Source: CAD feature listing. Evaluate the final solid. Frame: model axes, mm. Give positions to 0.01 mm unless a question says otherwise; leave off trailing zeros. One line per question, with ' | ' between items. Start each with the question number.
(1) Section A-A, the plane y = 5. State how many separate pieces and enclosed holes the cut face has, plus the area to 3 significant figures.
(2) Ray query, line 1 (Y direction, x = -20, z = 1.1); line 2 (Y direction, x = 72, z = 1.7). Return the intervals inside material, ascending. Write a range as [from, to].
(3) Pin query (flat end, axial travel): pin 1 (1 mm diameter, centred on y = 4.5, z = 2, fed in from -X). Return the tip coordinate at first contact, or that it passes through.
```python
from build123d import *

# Parameters (mm, degrees)
SALIENTE_EXTRUIR1_DEPTH = 3


with BuildPart() as part:
    # Croquis1 → Saliente-Extruir1 (new body)
    with BuildSketch(Plane.XY):
        Polygon((-150, 2.5), (-165, 2.5), (-165, -7.5), (-150, -7.5), (150, -7.5), (165, -7.5), (165, 2.5), (150, 2.5), (147.707897557, 7.5), (145, 2.5), (142.707897557, 7.5), (140, 2.5), (137.707897557, 7.5), (135, 2.5), (132.707897557, 7.5), (130, 2.5), (127.707897557, 7.5), (125, 2.5), (122.707897557, 7.5), (120, 2.5), (117.707897557, 7.5), (115, 2.5), (112.707897557, 7.5), (110, 2.5), (107.707897557, 7.5), (105, 2.5), (102.707897557, 7.5), (100, 2.5), (97.707897557, 7.5), (95, 2.5), (92.707897557, 7.5), (90, 2.5), (87.707897557, 7.5), (85, 2.5), (82.707897557, 7.5), (80, 2.5), (77.707897557, 7.5), (75, 2.5), (72.707897557, 7.5), (70, 2.5), (67.707897557, 7.5), (65, 2.5), (62.707897557, 7.5), (60, 2.5), (57.707897557, 7.5), (55, 2.5), (52.707897557, 7.5), (50, 2.5), (47.707897557, 7.5), (45, 2.5), (42.707897557, 7.5), (40, 2.5), (37.707897557, 7.5), (35, 2.5), (32.707897557, 7.5), (30, 2.5), (27.707897557, 7.5), (25, 2.5), (22.707897557, 7.5), (20, 2.5), (17.707897557, 7.5), (15, 2.5), (12.707897557, 7.5), (10, 2.5), (7.707897557, 7.5), (5, 2.5), (2.707897557, 7.5), (0, 2.5), (-2.292102443, 7.5), (-5, 2.5), (-7.292102443, 7.5), (-10, 2.5), (-12.292102443, 7.5), (-15, 2.5), (-17.292102443, 7.5), (-20, 2.5), (-22.292102443, 7.5), (-25, 2.5), (-27.292102443, 7.5), (-30, 2.5), (-32.292102443, 7.5), (-35, 2.5), (-37.292102443, 7.5), (-40, 2.5), (-42.292102443, 7.5), (-45, 2.5), (-47.292102443, 7.5), (-50, 2.5), (-52.292102443, 7.5), (-55, 2.5), (-57.292102443, 7.5), (-60, 2.5), (-62.292102443, 7.5), (-65, 2.5), (-67.292102443, 7.5), (-70, 2.5), (-72.292102443, 7.5), (-75, 2.5), (-77.292102443, 7.5), (-80, 2.5), (-82.292102443, 7.5), (-85, 2.5), (-87.292102443, 7.5), (-90, 2.5), (-92.292102443, 7.5), (-95, 2.5), (-97.292102443, 7.5), (-100, 2.5), (-102.292102443, 7.5), (-105, 2.5), (-107.292102443, 7.5), (-110, 2.5), (-112.292102443, 7.5), (-115, 2.5), (-117.292102443, 7.5), (-120, 2.5), (-122.292102443, 7.5), (-125, 2.5), (-127.292102443, 7.5), (-130, 2.5), (-132.292102443, 7.5), (-135, 2.5), (-137.292102443, 7.5), (-140, 2.5), (-142.292102443, 7.5), (-145, 2.5), (-147.292102443, 7.5), align=None)
    extrude(amount=SALIENTE_EXTRUIR1_DEPTH)


solid = part.part
```
Check sheet entries:
1) separate pieces: 60 | enclosed holes: 0 | area: 450 mm²
2) line 1: [-7.5, 2.5] | line 2: [-7.5, 6.19]
3) pin 1: x = -149.19
